Answer from the drawing. Dimensions are ordinates in mm from the lowest x, y and z of the part. A direction names the side the tool comes from. Coordinates: 2 decimals unless noted, no trailing zeros. Order: outer loops, then holes, each group sorted by start corner. A loop starts at its lowest first (then second) coordinate and runs counter-clockwise, first axis right, second up. Notation, with made-up numbers: (-37, 82.25) - (-18, 82.25) arc R13 ccw to (-18, 100.25) - close; hole circle Ø1 at (15.25, 37.5). An arc over 180 degrees is marked (long way). Answer as a JSON object with one key per item and string values. Group by question number.
1) Each of these flat-tipped pins is pushed along its axis until it touches: P1, Ø1.2, axis at x = 9, y = 6, coming from the +Z side (1 decimal); P2, Ø2, axis at x = 3.5, z = 16.5, coming from the -Y side; P3, Ø3, axis at y = 2, z = 13.5, coming from the -X side; P4, Ø3, axis at y = 5.5, z = 17.5, coming from the +X side. Where does it stop, or does it pass through?
2) Section C-C (z = 4) is taken. Give the vertices of the cut face in (x, y) (1 decimal).
3) Section A-A (z = 17) is taken. Give the vertices of the cut face in (x, y) (1 decimal).
4) The mould has two halves that part along Y. Classify the marked faces 4, 5 and 6: released by +Y, released by -Y, zero draft, split by the parting line, or undercut.
5) Section B-B (y = 8.5) is taken. Give the vertices of the cut face in (x, z) (1 decimal).
6) A tool of negligible diameter and unlimited length cuts with its end or side. For the marked faces 1, 2 and 3, from which of +Z, -Z, +X, -X, +Y, -Y can it reach the whole face along a straight path? Write none if from no direction.
7) Section D-D (z = 11.5) is taken. Give the vertices of the cut face in (x, y) (1 decimal).
8) Find the intervals of material crossed by line 1 along X through (y, z) = (6.75, 4.5) (1 decimal); line 2 along Z through (x, y) = (8.5, 8) (1 decimal); line 3 along X through (y, z) = (5.25, 20.75), in increasing order.
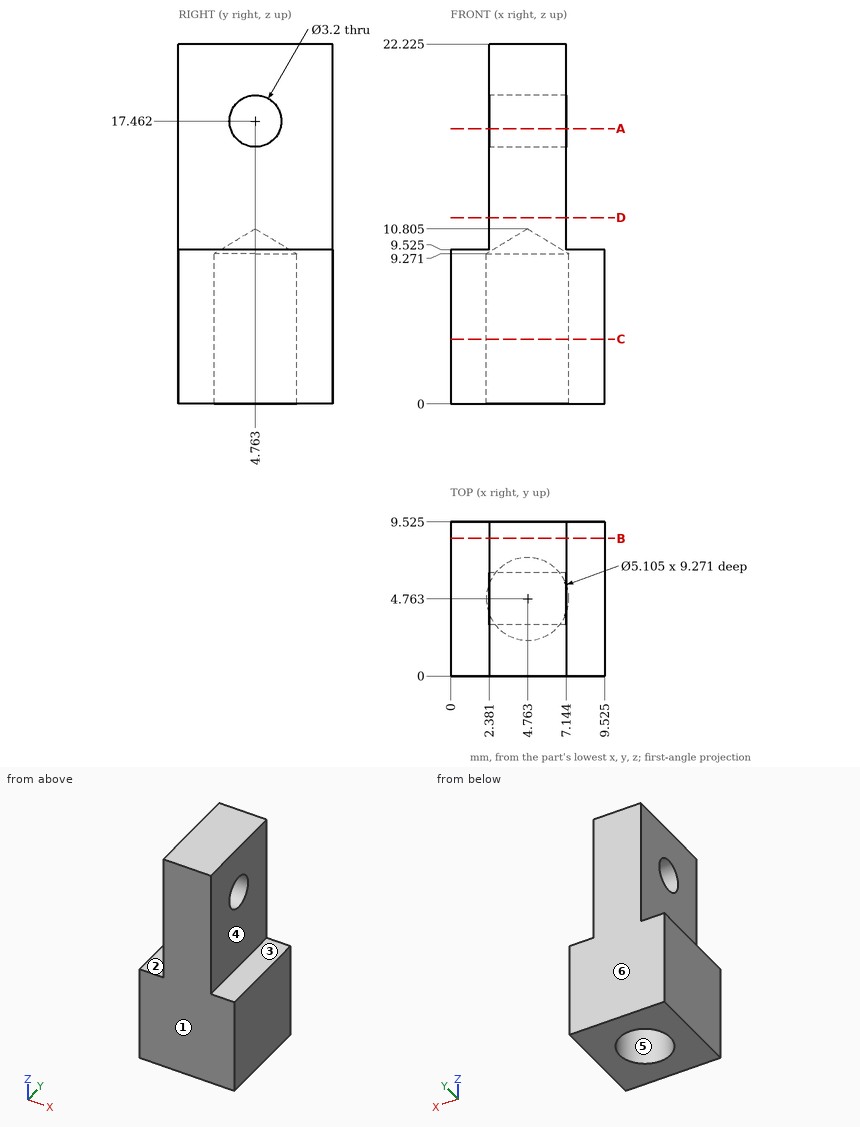
Report:
{
 "1": {"P1": "stops at z = 9.5", "P2": "stops at y = 0", "P3": "stops at x = 2.38", "P4": "stops at x = 7.14"},
 "2": {"outline": "(0, 0) - (9.5, 0) - (9.5, 9.5) - (0, 9.5) - close; hole circle Ø5.1 at (4.8, 4.8)"},
 "3": {"outline": "(2.4, 0) - (7.1, 0) - (7.1, 3.2) - (2.4, 3.2) - close; (2.4, 6.3) - (7.1, 6.3) - (7.1, 9.5) - (2.4, 9.5) - close"},
 "4": {"face 4": "zero draft", "face 5": "undercut", "face 6": "released by +Y"},
 "5": {"outline": "(0, 0) - (9.5, 0) - (9.5, 9.5) - (7.1, 9.5) - (7.1, 22.2) - (2.4, 22.2) - (2.4, 9.5) - (0, 9.5) - close"},
 "6": {"face 1": "+Z, -Z, +X, -X, -Y", "face 2": "+Z, -X, +Y, -Y", "face 3": "+Z, +X, +Y, -Y"},
 "7": {"outline": "(2.4, 0) - (7.1, 0) - (7.1, 9.5) - (2.4, 9.5) - close"},
 "8": {"line 1": "x = 0 to 3.2, 6.4 to 9.5", "line 2": "z = 0 to 9.5", "line 3": "x = 2.38 to 7.14"}
}
